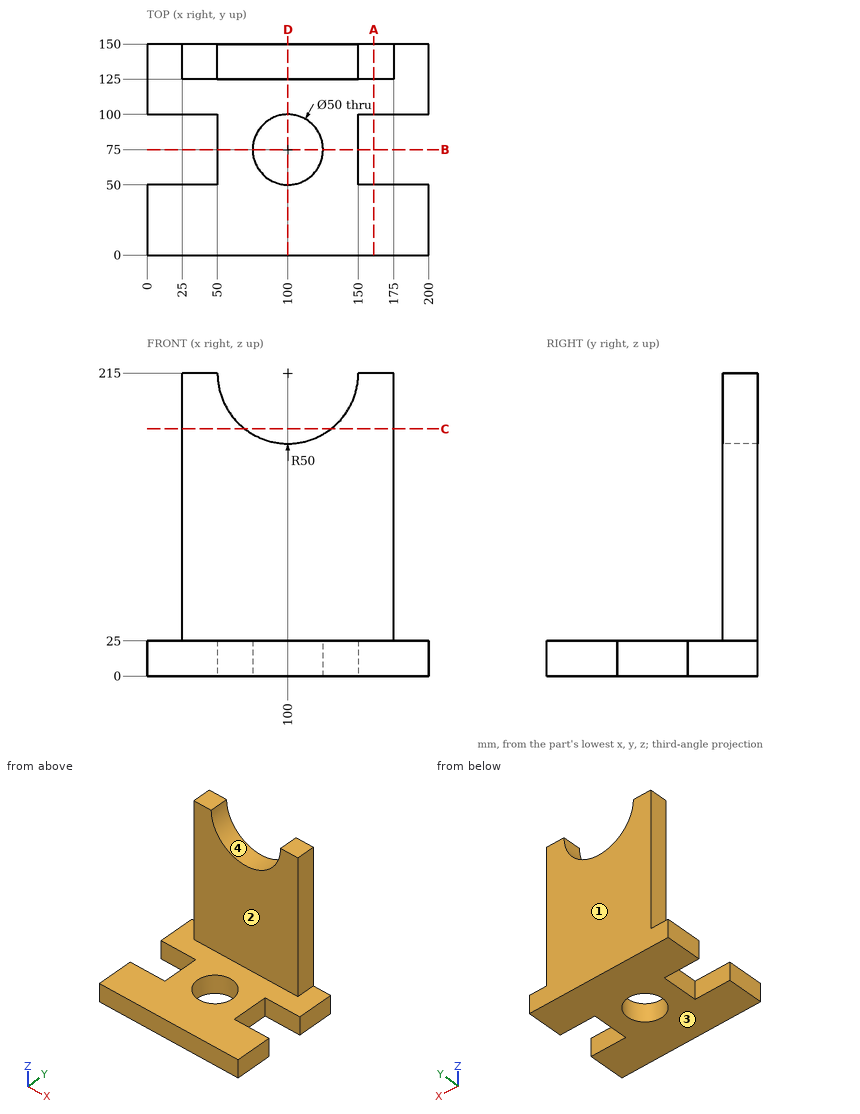
Here's the drawing with two shaded views (mm, measured from the low corner). I have some questions. A direction names the side the tool comes from. Coordinates: 2 decimals unless noted, no trailing zeros. Order: outer loops, then holes, each group sorted by start corner. A loop starts at its lowest first (then second) coordinate and runs counter-clockwise, first axis right, second up.
Q1. Suppose I cut it at B-B on y = 75. Please give me the cut outline in (x, z).
Q2. Suppose I cut it at D-D on x = 100. Please give me the cut outline in (y, z), and give its area (3 significant figures).
Q3. Which directions (+Z, -Z, +X, -X, +Y, -Y) give clear straight access to the entire face, cutting with the end or side of a thin tool? Please do the marked faces 1 and 2.
Q4. Suppose I cut it at A-A on x = 161. Please give me the cut outline in (y, z), and give its area (3 significant figures).
Q5. Please list where these lines run through material, in increasing order: L1, parallel to X at y = 75, z = 9.75; L2, parallel to Y at x = 100, z = 6; L3, parallel to X at y = 132, z = 28.
Q6. Will these pins go through, and if not, where does the flat tip stop? pin 1 (7.5 mm diameter, centred on y = 137.5, z = 76, fed in from +X); pin 2 (3 mm diameter, centred on x = 128, y = 62, fed in from +Z); pin 3 (3 mm diameter, centred on x = 153, y = 66, fed in from -Z); pin 4 (12.5 mm diameter, centred on y = 82.5, z = 15, fed in from -X).
Q7. Suppose I cut it at C-C on z = 175.5. Please give me the cut outline in (x, y).
Q8. Thinking about a two-plate mould opening in X: for the marked faces 3 and 4, which applies, released by +X, released by -X, zero draft, split by the parting line, or undercut?
Answer:
1. outline: (50, 0) - (75, 0) - (75, 25) - (50, 25) - close; (125, 0) - (150, 0) - (150, 25) - (125, 25) - close
2. outline: (0, 0) - (50, 0) - (50, 25) - (0, 25) - close; (100, 0) - (150, 0) - (150, 165) - (125, 165) - (125, 25) - (100, 25) - close
2. area: 6,000 mm2
3. face 1: +Z, -Z, +X, -X, +Y
3. face 2: +Z, +X, -X, -Y
4. outline: (0, 0) - (50, 0) - (50, 25) - (0, 25) - close; (100, 0) - (150, 0) - (150, 215) - (125, 215) - (125, 25) - (100, 25) - close
4. area: 7,250 mm2
5. L1: x = 50 to 75, 125 to 150
5. L2: y = 0 to 50, 100 to 150
5. L3: x = 25 to 175
6. pin 1: stops at x = 175
6. pin 2: stops at z = 25
6. pin 3: passes through
6. pin 4: stops at x = 50
7. outline: (25, 125) - (69.34, 125) - (69.34, 150) - (25, 150) - close; (130.66, 125) - (175, 125) - (175, 150) - (130.66, 150) - close
8. face 3: zero draft
8. face 4: undercut
